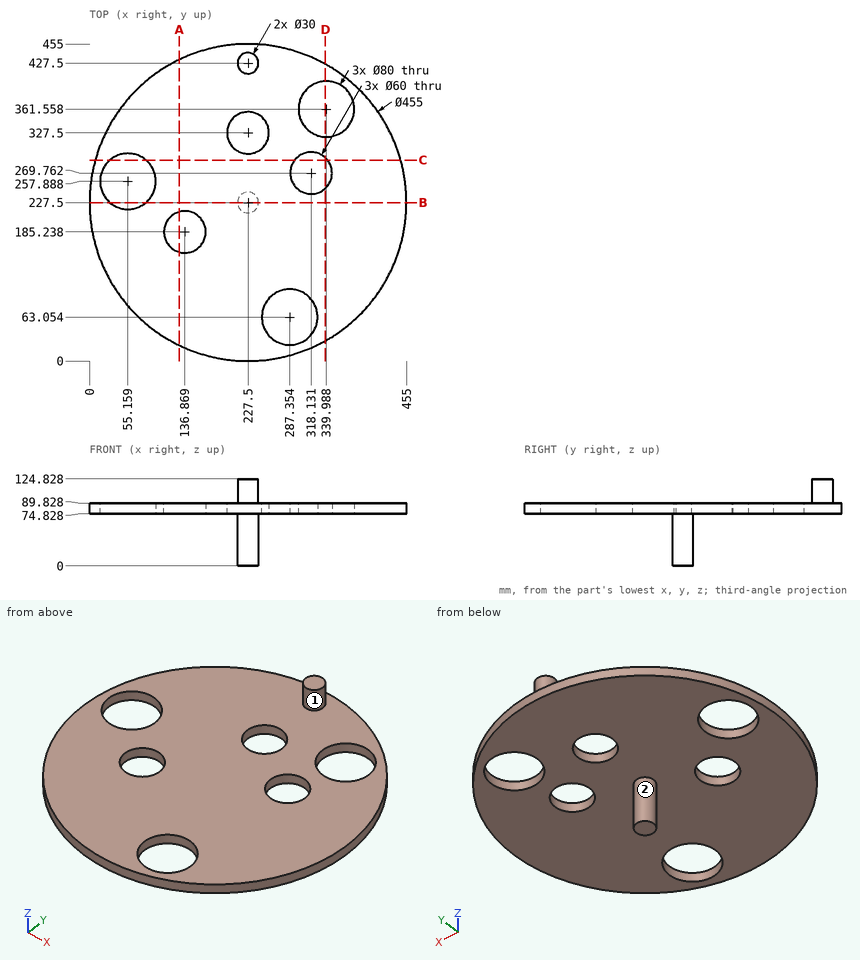
Answer from the drawing. Dimensions are ordinates in mm from the lowest x, y and z of the part. A direction names the side the tool comes from. Round coordinates to 2 decimals unless told otherwise and drop trailing zeros. Write each loop counter-clockwise with the first axis right and the second up, starting at its lowest first coordinate (ties: lowest second). Pieces come first, ordered by that corner, then holes.
1. The part is cut by section B-B, the plane y = 227.5. Determine the outline of the cut face in (x, z).
2. The part is cut by section C-C, the plane y = 288.5. Determine the outline of the cut face in (x, z).
3. Which of the six approach directions +Z, -Z, +X, -X, +Y, -Y give full straight-line access (tool end or side, diameter ignored) to the marked faces 1 and 2?
4. Given pin 1 Ø2 at (x, z) = (120, 75.5) entering from +Y; pin 2 Ø1.5 at (x, y) = (287.5, 313.5) entering from -Z; pin 3 Ø1.5 at (x, y) = (209.5, 194) entering from +Z, each flat-ended and moving along its own axis, determine where each tip first touches the part or whether it passes through.
5. The part is cut by section A-A, the plane x = 129. Determine the outline of the cut face in (y, z).
6. Straight lines are drawn through the part: L1, parallel to Z at x = 123.5, y = 157; L2, parallel to X at y = 208, z = 83 (1 decimal); L3, parallel to X at y = 236, z = 9. For each, find the intervals that lie inside material, in ascending order.
7. The part is cut by section D-D, the plane x = 338.5. Determine the outline of the cut face in (y, z) (1 decimal).
Values:
1. outline: (0, 74.83) - (29.15, 74.83) - (29.15, 89.83) - (0, 89.83) - close; (81.17, 74.83) - (212.5, 74.83) - (212.5, 0) - (242.5, 0) - (242.5, 74.83) - (455, 74.83) - (455, 89.83) - (81.17, 89.83) - close
2. outline: (8.33, 74.83) - (29.41, 74.83) - (29.41, 89.83) - (8.33, 89.83) - close; (80.91, 74.83) - (294.7, 74.83) - (294.7, 89.83) - (80.91, 89.83) - close; (341.56, 74.83) - (446.67, 74.83) - (446.67, 89.83) - (341.56, 89.83) - close
3. face 1: +Z
3. face 2: -Z
4. pin 1: stops at y = 428.53
4. pin 2: stops at z = 74.83
4. pin 3: stops at z = 89.83
5. outline: (22.43, 74.83) - (156.29, 74.83) - (156.29, 89.83) - (22.43, 89.83) - close; (214.19, 74.83) - (432.57, 74.83) - (432.57, 89.83) - (214.19, 89.83) - close
6. L1: z = 74.83 to 89.83
6. L2: x = 0.8 to 117.3, 156.4 to 454.2
6. L3: x = 215.14 to 239.86
7. outline: (28.9, 74.8) - (247.7, 74.8) - (247.7, 89.8) - (28.9, 89.8) - close; (291.8, 74.8) - (321.6, 74.8) - (321.6, 89.8) - (291.8, 89.8) - close; (401.5, 74.8) - (426.1, 74.8) - (426.1, 89.8) - (401.5, 89.8) - close
